from build123d import *

# Parameters (mm, degrees)
CUT_EXTRUDE1_DEPTH      = 51.305467894
CUT_EXTRUDE2_DEPTH      = 53.265868848
CUT_EXTRUDE2_DEPTH_BACK = 53.265868848
SKETCH6_R               = 3.852050009


with BuildPart() as part:
    # Sketch3 → Revolve1 (revolve)
    with BuildSketch(Plane.XY):
        with BuildLine():
            Line((0, 46.99), (0, 0))
            Line((0, 0), (12.7, 0))
            Line((12.7, 0), (12.7, 34.29))
            ThreePointArc((12.7, 34.29), (8.980256121, 43.270256121), (0, 46.99))
        make_face()
    revolve(axis=Axis((0, 46.99, 0), (0, -1, 0)))

    # Sketch4 → Cut-Extrude1 (cut, symmetric)
    with BuildSketch(Plane(origin=(0, 0, 0), x_dir=(0, 0, -1), z_dir=(1, 0, 0))):
        Polygon((-6.28327957, 45.326774794), (-6.35, 7.872595515), (-12.7, 7.872595515), (-15.471425878, 7.872595515), (-17.507867096, 7.199216011), (-21.88483387, 7.199216011), (-21.88483387, 45.326774794), align=None)
    cut_extrude1 = extrude(amount=CUT_EXTRUDE1_DEPTH, both=True, mode=Mode.SUBTRACT)

    # Mirror1: Cut-Extrude1 across plane
    add(cut_extrude1.mirror(Plane.XY), mode=Mode.SUBTRACT)

    # Sketch6 → Cut-Extrude2 (cut, two sides: drawn at the far end of the back side and taken through both)
    with BuildSketch(Plane(origin=(0, 0.011336761, 6.364003953), x_dir=(1, 0, 0), z_dir=(0, 0.0017813853062925587, 0.9999984133319366)).offset(-CUT_EXTRUDE2_DEPTH_BACK)):
        with Locations(Location((0, 32.687978784, 0), (0, 0, 270))):
            Circle(SKETCH6_R)
    extrude(amount=CUT_EXTRUDE2_DEPTH + CUT_EXTRUDE2_DEPTH_BACK, mode=Mode.SUBTRACT)


solid = part.part
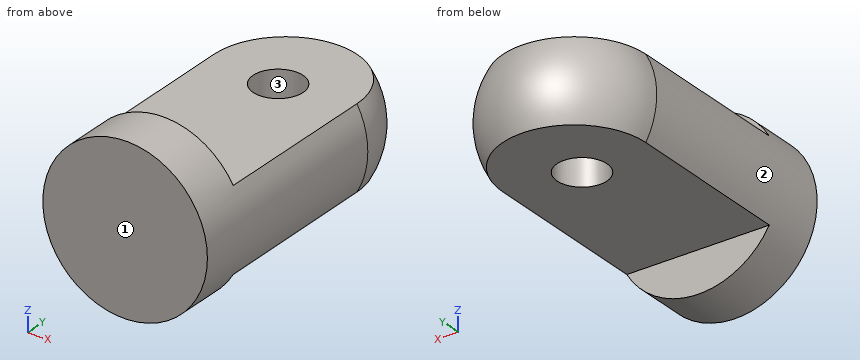
Design review of the part built by this model. Coordinates are the model's own, in mm. Face numbers are marked on the shaded views. Coordinates: 2 decimals unless noted, no trailing zeros. Write each loop counter-clockwise with the first axis right and the second up, starting at its lowest first coordinate (ties: lowest second). Pieces come first, ordered by that corner, then holes. Notation, with made-up numbers: (-0.75, 62.25) - (35.25, 62.25) arc R20 cw to (35.25, 99.25) - close; hole circle Ø2 at (86, -1.75). An arc over 180 degrees is marked (long way). Use one line per item in the form item = value.
Q1. Consider section A-A (x = 0). Write out the cut boundary in (y, z), plus the area to 3 significant figures.
Taken from the geometry:
outline = (0, -12.7) - (7.87, -12.7) - (7.87, -6.35) - (28.82, -6.31) - (28.85, 6.31) - (7.87, 6.35) - (7.87, 12.7) - (0, 12.7) - close; (36.53, -6.3) - (45.33, -6.28) arc R12.7 ccw to (45.33, 6.28) - (36.55, 6.3) - close
area = 590 mm^2
Q2. Insertion check: pin 1 Ø2 at (x, z) = (-3.5, -8.5) entering from +Y; pin 2 Ø1.5 at (y, z) = (37.5, 5.5) entering from +X; pin 3 Ø4 at (y, z) = (14, 6) entering from -X. Each pin has a flat end and moves straight along its axis. Give the tip position at first contact, or say it passes through.
Taken from the geometry:
pin_1 = 7.87
pin_2 = 11.39
pin_3 = -12.05
Q3. Consider section B-B (x = 9). Write out the cut boundary in (y, z), plus the area to 3 significant figures.
Taken from the geometry:
outline = (0, -8.96) - (7.87, -8.96) - (7.87, -6.35) - (40.67, -6.29) arc R8.96 ccw to (40.67, 6.29) - (7.87, 6.35) - (7.87, 8.96) - (0, 8.96) - close
area = 578 mm^2
Q4. Consider section D-D (z = 8.25). Write out the cut boundary in (x, y), plus the area to 3 significant figures.
Taken from the geometry:
outline = (-9.66, 0) - (9.66, 0) - (9.66, 7.87) - (-9.66, 7.87) - close
area = 152 mm^2
Q5. For probe 1 along Z at (x, y) = (-2.75, 41); probe 2 along Y at (x, z) = (6, 10.75); probe 3 along Y at (x, z) = (9.5, 1.5), list the stretches that pass through material, from the lowest coordinate up.
Taken from the geometry:
probe_1 = -6.29 to 6.29
probe_2 = 0 to 7.87
probe_3 = 0 to 42.58
Q6. Consider section C-C (y = 13.5). Write out the cut boundary in (x, z), plus the area to 3 significant figures.
Taken from the geometry:
outline = (-11, -6.34) - (11, -6.34) arc R12.7 ccw to (11, 6.34) - (-11, 6.34) arc R12.7 ccw to start
area = 308 mm^2
Q7. The part is to be moulded in two halves that separate along X. For the marked faces 1, 2 and 3, say which applies: +X half, -X half, draft (parallel to the pull), parting line (faces both ways), or undercut.
Taken from the geometry:
face_1 = draft
face_2 = parting line
face_3 = undercut
